Study the drawing (mm; zero at the part's minimum x, y, z) and answer. A direction names the side the tool comes from. Give positions to 0.01 mm unless a question says otherwise; leave off trailing zeros. Write each loop counter-clockwise with the first axis right and the second up, starting at its lowest first coordinate (ties: lowest second). Pieces come first, ordered by that corner, then holes. Notation, with made-up numbers: (1.5, 5.25) -> (14.5, 5.25) arc R23 ccw to (14.5, 36.25) -> close; hole circle Ø2 at (52.25, 9). An arc over 180 degrees is marked (long way). One line per question, with ' | ' between items.
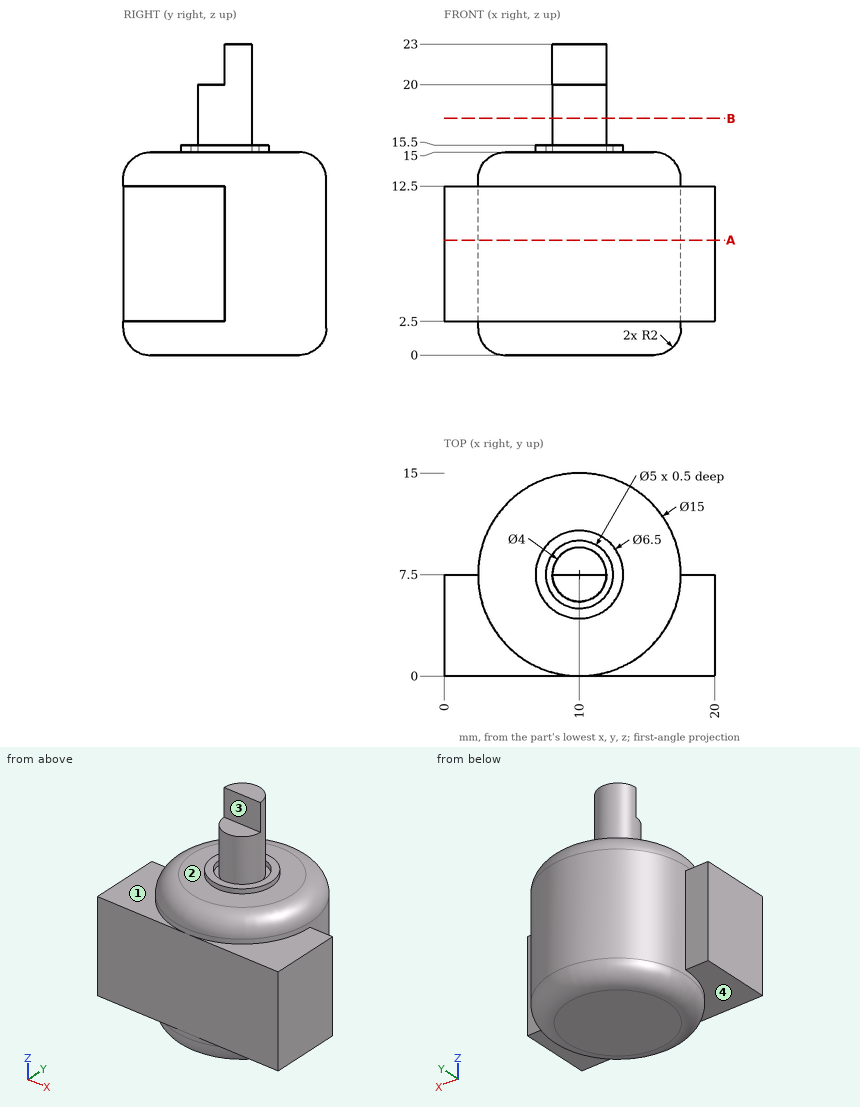
Item 1: Flat-ended cylindrical pins translate along their axes: pin 1 (8 mm diameter, centred on x = 16.5, y = 3.5, fed in from +Z); pin 2 (4 mm diameter, centred on x = 12.5, y = 11, fed in from +Z); pin 3 (0.6 mm diameter, centred on x = 9, y = 6.5, fed in from +Z). Find the tip coordinate at first contact, or state that the pin passes through.
Answers below:
pin 1: z = 15 | pin 2: z = 15.5 | pin 3: z = 20
Item 2: Find section A-A (z = 8.5). Write down the section's boundary in (x, y), then the cut area to 3 significant figures.
Answers below:
outline: (0, 0) -> (20, 0) -> (20, 7.5) -> (17.5, 7.5) arc R7.5 ccw to (2.5, 7.5) -> (0, 7.5) -> close | area: 238 mm²
Item 3: Consider line 1 (Y direction, x = 10, z = 15.3); line 2 (Z direction, x = 13.75, y = 5); line 3 (Y direction, x = 1.5, z = 6.5). Determine where each line is inside the solid, lowest interval first. Write a range as [from, to].
Answers below:
line 1: [4.25, 5], [5.5, 9.5], [10, 10.75] | line 2: [0, 15] | line 3: [0, 7.5]
Item 4: Find section B-B (z = 17.5). Write down the section's boundary in (x, y), then the cut area to 3 significant figures.
Answers below:
outline: circle Ø4 at (10, 7.5) | area: 12.6 mm²
Item 5: A tool of negligible diameter and unlimited length cuts with its end or side. For the marked faces 1, 2, 3 and 4, from which of +Z, -Z, +X, -X, +Y, -Y can it reach the whole face along a straight path? Write none if from no direction.
Answers below:
face 1: +Z, -X, -Y | face 2: +Z | face 3: +Z, +X, -X, -Y | face 4: -Z, -X, -Y
